```python
from build123d import *

# Parameters (mm, degrees)
CROQUIS1_W              = 60
CROQUIS1_H              = 60
SALIENTE_EXTRUIR1_DEPTH = 10
REDONDEO1_R             = 5
CROQUIS2_R              = 4
SALIENTE_EXTRUIR2_DEPTH = 125
CROQUIS3_W              = 60
CROQUIS3_H              = 60
CROQUIS3_R              = 4
SALIENTE_EXTRUIR4_DEPTH = 10
REDONDEO2_R             = 5


with BuildPart() as part:
    # Croquis1 → Saliente-Extruir1 (new body)
    with BuildSketch(Plane.XY):
        Rectangle(CROQUIS1_W, CROQUIS1_H)
        Polygon((42.5, -30), (30, -30), (-30, -30), (-42.5, -30), (-42.5, -35), (42.5, -35), align=None)
    extrude(amount=SALIENTE_EXTRUIR1_DEPTH)

    # Redondeo1
    redondeo1_edges = [part.edges().sort_by_distance(p)[0] for p in [
        (30, 30, 5),
        (-30, 30, 5),
    ]]
    fillet(redondeo1_edges, radius=REDONDEO1_R)

    # Croquis2 → Saliente-Extruir2 (add)
    with BuildSketch(Plane(origin=(0, 0, 0), x_dir=(-1, 0, 0), z_dir=(0, 0, -1))):
        with Locations(Location((-20, 20, 0), (0, 0, 180))):
            Circle(CROQUIS2_R)
        with Locations(Location((20, 20, 0), (0, 0, 180))):
            Circle(CROQUIS2_R)
    extrude(amount=SALIENTE_EXTRUIR2_DEPTH)

    # Croquis3 → Saliente-Extruir4 (add)
    # profile 1 of 3: a face of its own
    with BuildSketch(Plane(origin=(0, 0, -125), x_dir=(-1, 0, 0), z_dir=(0, 0, -1))):
        Rectangle(CROQUIS3_W, CROQUIS3_H)
        with Locations(Location((20, 20, 0), (0, 0, 180))):
            Circle(CROQUIS3_R, mode=Mode.SUBTRACT)
    # profile 2 of 3: a face of its own
    with BuildSketch(Plane(origin=(0, 0, -125), x_dir=(-1, 0, 0), z_dir=(0, 0, -1))):
        Polygon((30, -30), (-30, -30), (-42.5, -30), (-42.5, -35), (42.5, -35), (42.5, -30), align=None)
    # profile 3 of 3: a face of its own
    with BuildSketch(Plane(origin=(0, 0, -125), x_dir=(-1, 0, 0), z_dir=(0, 0, -1))):
        with Locations(Location((20, 20, 0), (0, 0, 180))):
            Circle(CROQUIS3_R)
    extrude(amount=SALIENTE_EXTRUIR4_DEPTH)

    # Redondeo2
    redondeo2_edges = [part.edges().sort_by_distance(p)[0] for p in [
        (-30, 30, -130),
        (30, 30, -130),
    ]]
    fillet(redondeo2_edges, radius=REDONDEO2_R)


solid = part.part
```
Source: CAD feature listing. Evaluate the final solid. Frame: model axes, mm. A direction names the side the tool comes from. Give positions to 0.01 mm unless a question says otherwise; leave off trailing zeros. Order: outer loops, then holes, each group sorted by start corner. A loop starts at its lowest first (then second) coordinate and runs counter-clockwise, first axis right, second up. Notation, with made-up numbers: (-18.75, 46.5) -> (-4.75, 46.5) arc R13 cw to (-4.75, 51.5) -> close; hole circle Ø5 at (23.5, 57.5). An arc over 180 degrees is marked (long way). Use a Markdown table: item, result.
Q1. Access query for faces 4 (the face through (-1, -2, 10)), 5 (the face through (19.479, 16.034, -61.625)), 6 (the face through (-36, -30, -130)), 7 (the face through (36, -30, -130)), 8 (the face through (0, 30, -130)). Directions: +Z, -Z, +X, -X, +Y, -Y. A direction counts if a zero-diameter tool reaches every point of the face in a straight line with its end or side. Return the directions, or none.
A:
| item | result |
|---|---|
| face 4 | +Z, +X, -X, +Y, -Y |
| face 5 | none |
| face 6 | +Z, -Z, -X, +Y |
| face 7 | +Z, -Z, +X, +Y |
| face 8 | +Z, -Z, +X, -X, +Y |
Q2. Pull-direction query (Z, two-part tool) for faces 1 (the face through (-42.5, -32, 5)), 2 (the face through (1, -2, -135)), 3 (the face through (-1, -2, 0)); classes: +Z half, -Z half, draft (parallel to the pull), parting line (faces both ways), or undercut.
A:
| item | result |
|---|---|
| face 1 | draft |
| face 2 | -Z half |
| face 3 | undercut |
Q3. Section C-C (x = -20). Return the cut outline in (y, z).
A:
| item | result |
|---|---|
| outline | (-35, -135) -> (30, -135) -> (30, -125) -> (24, -125) -> (24, 0) -> (30, 0) -> (30, 10) -> (-35, 10) -> (-35, 0) -> (16, 0) -> (16, -125) -> (-35, -125) -> close |
Q4. First-contact query: P1, Ø5, axis at y = 8, z = -128, coming from the +X side; P2, Ø12, axis at x = 10.5, z = -113, coming from the -Y side; P3, Ø8, axis at y = 2.5, z = 5, coming from the -X side. Flat tips, straight axial feed; report the tip coordinate or a pass-through.
A:
| item | result |
|---|---|
| P1 | x = 30 |
| P2 | y = 18.06 |
| P3 | x = -30 |
Q5. Material intervals for line 1 (Z direction, x = 21, y = -18); line 2 (X direction, y = 20, z = -102); line 3 (X direction, y = -27.5, z = 0.5), sorted ascending. Write a range as [from, to].
A:
| item | result |
|---|---|
| line 1 | [-135, -125], [0, 10] |
| line 2 | [-24, -16], [16, 24] |
| line 3 | [-30, 30] |
Q6. Section B-B (y = 5.5). Return the cut outline in (x, z).
A:
| item | result |
|---|---|
| outline | (-30, -135) -> (30, -135) -> (30, -125) -> (-30, -125) -> close; (-30, 0) -> (30, 0) -> (30, 10) -> (-30, 10) -> close |
Q7. Section A-A (x = -34). Return the cut outline in (y, z), and give its area (3 significant figures).
A:
| item | result |
|---|---|
| outline | (-35, -135) -> (-30, -135) -> (-30, -125) -> (-35, -125) -> close; (-35, 0) -> (-30, 0) -> (-30, 10) -> (-35, 10) -> close |
| area | 100 mm^2 |
Q8. Section D-D (z = -59). Return the cut outline in (x, y), and give its area (3 significant figures).
A:
| item | result |
|---|---|
| outline | circle Ø8 at (-20, 20); circle Ø8 at (20, 20) |
| area | 101 mm^2 |
